Source: three-view drawing plus pictorial views. Frame: mm from the lowest corner of the part. A direction names the side the tool comes from. Round coordinates to 2 decimals unless told otherwise and drop trailing zeros. Write each loop counter-clockwise with the first axis right and the second up, starting at its lowest first coordinate (ties: lowest second). Pieces come first, ordered by that corner, then holes. Notation, with made-up numbers: (-3, 38.5) -> (37, 38.5) arc R23 cw to (37, 51.5) -> close; hole circle Ø7 at (-7, 7). An arc over 180 degrees is marked (long way). Put each result on its own line as item: value.
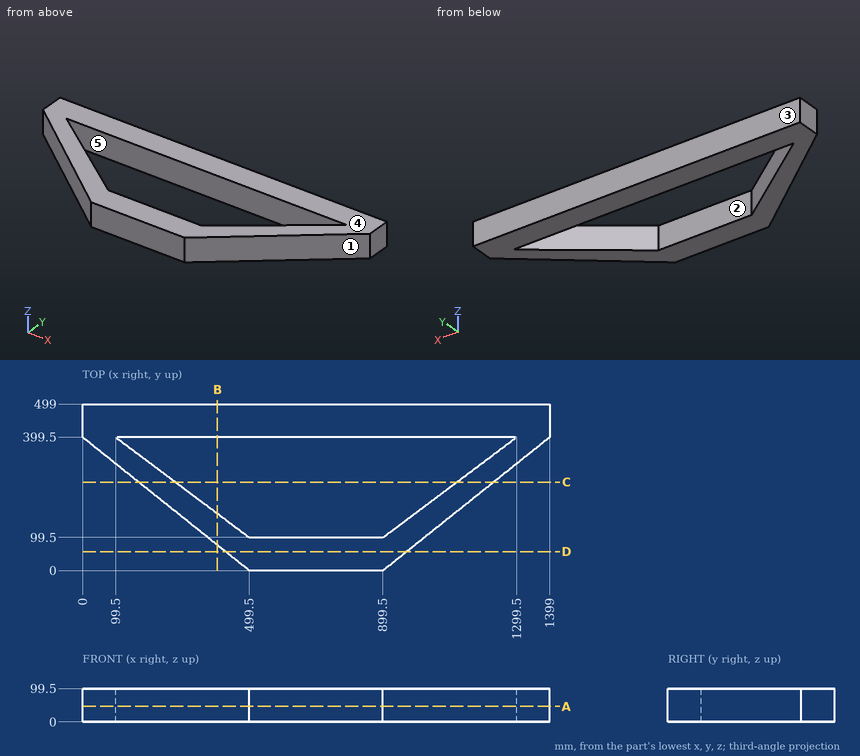
Q1. Cut plane A-A on z = 46.5. Output: boundary loops of the cut face in (x, y), and give its area (3 significant figures).
Ans:
outline: (0, 399.5) -> (499.5, 0) -> (899.5, 0) -> (1399, 399.5) -> (1399, 499) -> (0, 499) -> close; hole (99.5, 399.5) -> (499.5, 99.5) -> (899.5, 99.5) -> (1299.5, 399.5) -> close
area: 259,000 mm^2
Q2. Cut plane C-C on y = 265. Output: boundary loops of the cut face in (x, z), and give its area (3 significant figures).
Ans:
outline: (168.17, 0) -> (278.83, 0) -> (278.83, 99.5) -> (168.17, 99.5) -> close; (1120.17, 0) -> (1230.83, 0) -> (1230.83, 99.5) -> (1120.17, 99.5) -> close
area: 22,000 mm^2
Q3. Pin query (flat end, axial travel): pin 1 (1 mm diameter, centred on x = 233, z = 45, fed in from -Y); pin 2 (4 mm diameter, centred on y = 154.5, z = 62.5, fed in from -X); pin 3 (1 mm diameter, centred on y = 106.5, z = 88, fed in from -X). Return the tip coordinate at first contact, or that it passes through.
Ans:
pin 1: stops at y = 212.75
pin 2: stops at x = 303.83
pin 3: stops at x = 365.72
Q4. Cut plane D-D on y = 57. Output: boundary loops of the cut face in (x, z).
Ans:
outline: (428.23, 0) -> (970.77, 0) -> (970.77, 99.5) -> (428.23, 99.5) -> close
Q5. Draft query along X for the marked faces 1, 2 and 3. Return one class per face: +X half, -X half, draft (parallel to the pull), parting line (faces both ways), or undercut.
Ans:
face 1: +X half
face 2: undercut
face 3: draft
Q6. Material intervals for line 1 (Y direction, x = 775, z = 72); line 2 (Y direction, x = 1116, z = 48.5) (3 decimals); line 3 (X direction, y = 187, z = 44.5), sorted ascending. Write a range as [from, to].
Ans:
line 1: y = [0, 99.5], [399.5, 499]
line 2: y = [173.157, 261.875], [399.5, 499]
line 3: x = [265.69, 382.83], [1016.17, 1133.31]
Q7. Cut plane B-B on x = 404. Output: boundary loops of the cut face in (y, z) (3 decimals), and give its area (3 significant figures).
Ans:
outline: (76.381, 0) -> (171.125, 0) -> (171.125, 99.5) -> (76.381, 99.5) -> close; (399.5, 0) -> (499, 0) -> (499, 99.5) -> (399.5, 99.5) -> close
area: 19,300 mm^2
Q8. Reachability of the marked faces 4 and 5 from +Z, -Z, +X, -X, +Y, -Y: full face, straight path, thin tool, end or side. Return the list, or none.
Ans:
face 4: +Z, +X, -X, +Y, -Y
face 5: +Z, -Z
